Answer from the drawing. Dimensions are ordinates in mm from the lowest x, y and z of the part. Coordinates: 2 decimals unless noted, no trailing zeros. Write each loop counter-clockwise with the first axis right and the second up, starting at its lowest first coordinate (ties: lowest second). Pieces come first, ordered by that corner, then holes. Notation, with made-up numbers: (45.5, 85) - (60.5, 85) arc R29 cw to (60.5, 122) - close; hole circle Ø1 at (87, 52). An arc over 180 degrees is marked (long way). Answer as a JSON object with one key per item and string values. Group by question number.
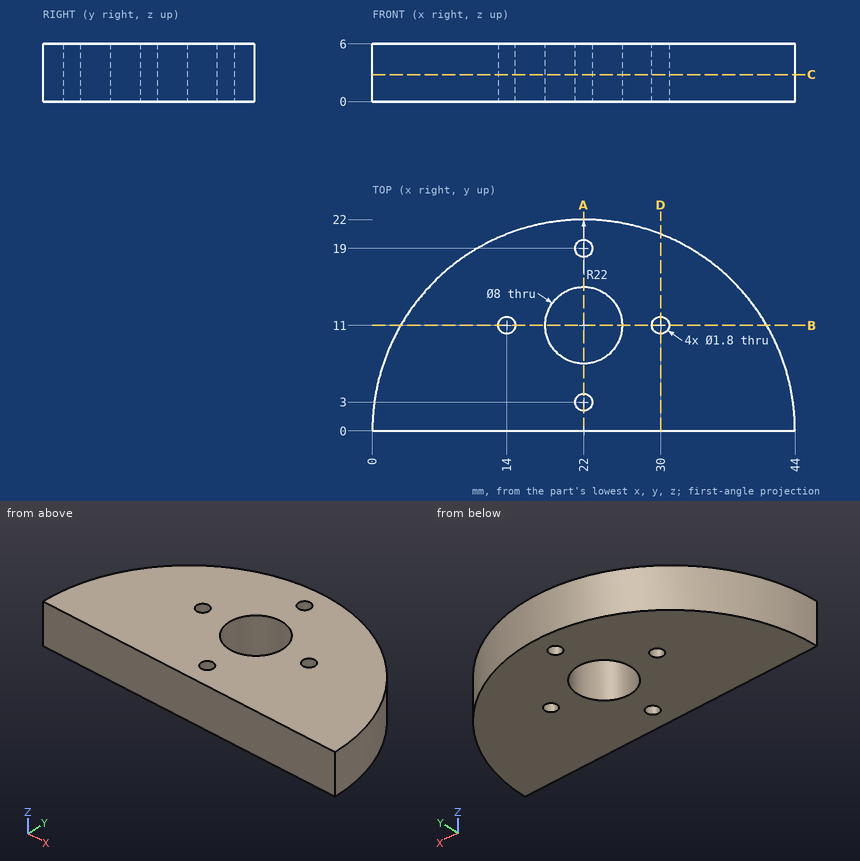
Q1. Consider L1, parallel to Y at x = 22, z = 1.4; L2, parallel to X at y = 10.75, z = 2.65; L3, parallel to Y at x = 29.5, z = 5.35. Determine where each line is inside the solid, lowest interval first. Write a range as from..to.
Q2. Flat-ended cylindrical pins translate along their axes: pin 1 Ø1 at (y, z) = (10.5, 2.5) entering from +X; pin 2 Ø3 at (y, z) = (8.5, 5) entering from +X. Find the tip coordinate at first contact, or state that the pin passes through.
Q3. Section C-C on z = 2.8 is taken. Determine the outline of the cut face in (x, y).
Q4. Section A-A on x = 22 is taken. Determine the outline of the cut face in (y, z).
Q5. Section D-D on x = 30 is taken. Determine the outline of the cut face in (y, z).
Q6. Section B-B on y = 11 is taken. Determine the outline of the cut face in (x, z).
Numbers:
{
 "1": {"L1": "y = 0..2.1, 3.9..7, 15..18.1, 19.9..22", "L2": "x = 2.81..13.14, 14.86..18.01, 25.99..29.14, 30.86..41.19", "L3": "y = 0..10.25, 11.75..20.68"},
 "2": {"pin 1": "stops at x = 41.6", "pin 2": "stops at x = 42.86"},
 "3": {"outline": "(0, 0) - (44, 0) arc R22 ccw to start; hole circle Ø1.8 at (14, 11); hole circle Ø8 at (22, 11); hole circle Ø1.8 at (22, 3); hole circle Ø1.8 at (22, 19); hole circle Ø1.8 at (30, 11)"},
 "4": {"outline": "(0, 0) - (2.1, 0) - (2.1, 6) - (0, 6) - close; (3.9, 0) - (7, 0) - (7, 6) - (3.9, 6) - close; (15, 0) - (18.1, 0) - (18.1, 6) - (15, 6) - close; (19.9, 0) - (22, 0) - (22, 6) - (19.9, 6) - close"},
 "5": {"outline": "(0, 0) - (10.1, 0) - (10.1, 6) - (0, 6) - close; (11.9, 0) - (20.49, 0) - (20.49, 6) - (11.9, 6) - close"},
 "6": {"outline": "(2.95, 0) - (13.1, 0) - (13.1, 6) - (2.95, 6) - close; (14.9, 0) - (18, 0) - (18, 6) - (14.9, 6) - close; (26, 0) - (29.1, 0) - (29.1, 6) - (26, 6) - close; (30.9, 0) - (41.05, 0) - (41.05, 6) - (30.9, 6) - close"}
}
